Part model, mm, in its own coordinate system. Face numbers are marked on the shaded views. A direction names the side the tool comes from. Round coordinates to 2 decimals unless told otherwise and drop trailing zeros. Write each loop counter-clockwise with the first axis right and the second up, starting at its lowest first coordinate (ties: lowest second). Pieces come first, ordered by that corner, then holes. Notation, with made-up numbers: (35.25, 4.25) -> (80.25, 4.25) arc R17 cw to (80.25, 24.25) -> close; hole circle Ø6 at (87.5, 1.25). An arc over 180 degrees is marked (long way). Return JSON: item names as keys, results as strings. Group by question number.
```python
from build123d import *

# Parameters (mm, degrees)
SKETCH1_R                    = 4.572
SKETCH1_R_2                  = 1.397
SKETCH1_R_3                  = 3.175
BOSS_EXTRUDE1_DEPTH          = 6.35
F_3_8_0_375_DIAMETER_SLOT1_D = 9.525
SKETCH6_W                    = 9.906
SKETCH6_H                    = 38.1
BOSS_EXTRUDE2_DEPTH          = 76.2
SKETCH7_R                    = 1.397
SKETCH7_R_2                  = 1.7859375
CUT_EXTRUDE1_DEPTH           = 107.68
CUT_EXTRUDE2_DEPTH           = 10.16


with BuildPart() as part:
    # Sketch1 → Boss-Extrude1 (new body)
    with BuildSketch(Plane(origin=(0, 0, 0), x_dir=(1, 0, 0), z_dir=(0, 1, 0))):
        with BuildLine():
            Line((-53.34, 57.15), (53.34, 57.15))
            Line((53.34, 57.15), (53.34, -57.15))
            ThreePointArc((53.34, -57.15), (0, -110.49), (-53.34, -57.15))
            Line((-53.34, -57.15), (-53.34, 57.15))
        make_face()
        Circle(SKETCH1_R, mode=Mode.SUBTRACT)
        with Locations((-12.7, -12.7)):
            Circle(SKETCH1_R_2, mode=Mode.SUBTRACT)
        with Locations((-12.7, 12.7)):
            Circle(SKETCH1_R_2, mode=Mode.SUBTRACT)
        with Locations((12.7, 12.7)):
            Circle(SKETCH1_R_2, mode=Mode.SUBTRACT)
        with Locations((12.7, -12.7)):
            Circle(SKETCH1_R_2, mode=Mode.SUBTRACT)
        with Locations((0, -93.791156658)):
            Circle(SKETCH1_R_3, mode=Mode.SUBTRACT)
    extrude(amount=BOSS_EXTRUDE1_DEPTH)

    # 3/8 (0.375) Diameter Slot1 (through all)
    with Locations(Plane(origin=(0, 6.35, 0), x_dir=(1, 0, 0), z_dir=(0, 1, 0))):
        with Locations((0, 0)):
            Hole(F_3_8_0_375_DIAMETER_SLOT1_D / 2)

    # Sketch6 → Boss-Extrude2 (add)
    with BuildSketch(Plane(origin=(0, 6.35, 0), x_dir=(1, 0, 0), z_dir=(0, 1, 0))):
        with Locations((-48.387, 0)):
            Rectangle(SKETCH6_W, SKETCH6_H)
        with Locations((48.387, 0)):
            Rectangle(SKETCH6_W, SKETCH6_H)
    extrude(amount=BOSS_EXTRUDE2_DEPTH)

    # Sketch7 → Cut-Extrude1 (cut, through all)
    with BuildSketch(Plane.ZY.offset(53.34)):
        with Locations((-9.906, 63.455207007)):
            Circle(SKETCH7_R)
        with Locations((0, 63.5)):
            Circle(SKETCH7_R_2)
        with Locations((-7.036273203, 70.472926346)):
            Circle(SKETCH7_R)
        with Locations((-0.044792993, 73.406)):
            Circle(SKETCH7_R)
        with Locations((6.972926346, 70.536273203)):
            Circle(SKETCH7_R)
        with Locations((9.906, 63.544792993)):
            Circle(SKETCH7_R)
        with Locations((7.036273203, 56.527073654)):
            Circle(SKETCH7_R)
        with Locations((0.044792993, 53.594)):
            Circle(SKETCH7_R)
        with Locations((-6.972926346, 56.463726797)):
            Circle(SKETCH7_R)
    extrude(amount=-CUT_EXTRUDE1_DEPTH, mode=Mode.SUBTRACT)

    # Sketch8 → Cut-Extrude2 (cut)
    with BuildSketch(Plane(origin=(0, 6.35, 0), x_dir=(1, 0, 0), z_dir=(0, 1, 0))):
        Polygon((29.925449695, 49.207255953), (20.005730679, 57.103391791), (20.005730679, 41.311120115), align=None)
        Polygon((29.925449695, 49.207255953), (20.005730679, 41.311120115), (39.84516871, 41.311120115), align=None)
        Polygon((39.84516871, 41.311120115), (39.84516871, 57.103391791), (29.925449695, 49.207255953), align=None)
        Polygon((39.84516871, 57.103391791), (20.005730679, 57.103391791), (29.925449695, 49.207255953), align=None)
    extrude(amount=-CUT_EXTRUDE2_DEPTH, mode=Mode.SUBTRACT)


solid = part.part
```
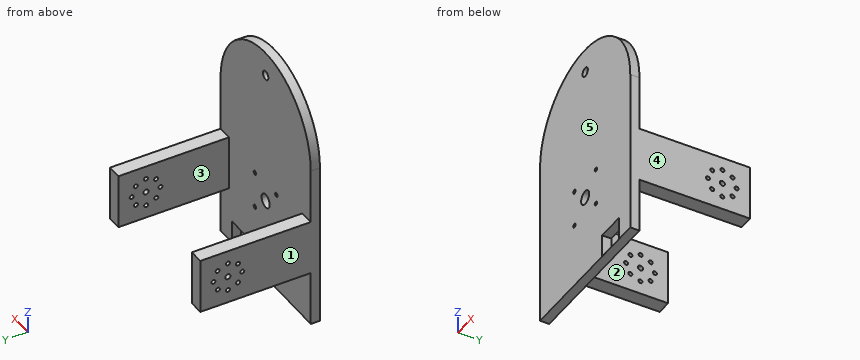
Item 1: Cut at B-B (y = 39.5). Write the cut outline in (x, z), then the cut area to 3 significant figures.
Item 2: Cut at D-D (x = -40). Write the cut outline in (y, z), then the cut area to 3 significant figures.
Item 3: Wall check: L1, parallel to Y at x = -46, z = 0; L2, parallel to X at y = 31, z = 3; L3, parallel to X at y = 4, z = 12. Give the ranges that are in metal, low to high.
Item 4: Two-plate mould, pull along X, no slides. Class the marked faces 3, 4 and 5: released by +X, released by -X, zero draft, split by the parting line, or undercut.
Item 5: Cut at C-C (z = -39). Write the cut outline in (x, y), then the cut area to 3 significant figures.
Item 6: Which spindle directions (+Z, -Z, +X, -X, +Y, -Y) get a long thin tool onto all of the face, cutting with end or side? Do the marked faces 1 and 2. Say none if no direction does.
Item 7: Cut at A-A (x = 0). Write the cut outline in (y, z), then the cut area to 3 significant figures.
Item 8: Flat gauge pins, fed straight in: P1, Ø8, axis at x = 46.5, y = 50.5, coming from the +Z side; P2, Ø12, axis at x = -4, y = 9, coming from the +Z side; P3, Ø1, axis at x = -27.5, z = 32.5, coming from the +Y side. Where does each tip first touch, or does it go through?
Checks:
{
 "1": {"outline": "(-53.34, -19.05) -> (-43.43, -19.05) -> (-43.43, 19.05) -> (-53.34, 19.05) -> close; (43.43, -19.05) -> (53.34, -19.05) -> (53.34, 19.05) -> (43.43, 19.05) -> close", "area": "755 mm2"},
 "2": {"outline": "(0, -57.15) -> (6.35, -57.15) -> (6.35, 92.44) -> (0, 92.44) -> close", "area": "950 mm2"},
 "3": {"L1": "y = 0 to 52.2, 54.99 to 61.71, 65.29 to 72.01, 74.8 to 82.55", "L2": "x = -53.34 to -43.43, 43.43 to 53.34", "L3": "x = -53.34 to -13.91, -11.49 to 11.49, 13.91 to 53.34"},
 "4": {"face 3": "undercut", "face 4": "released by +X", "face 5": "zero draft"},
 "5": {"outline": "(-53.34, 0) -> (53.34, 0) -> (53.34, 6.35) -> (-53.34, 6.35) -> close", "area": "677 mm2"},
 "6": {"face 1": "+Z, -Z, -X, +Y, -Y", "face 2": "+Z, -Z, +Y"},
 "7": {"outline": "(0, -57.15) -> (6.35, -57.15) -> (6.35, -4.76) -> (0, -4.76) -> close; (0, 4.76) -> (6.35, 4.76) -> (6.35, 90.62) -> (0, 90.62) -> close; (0, 96.97) -> (6.35, 96.97) -> (6.35, 110.49) -> (0, 110.49) -> close", "area": "964 mm2"},
 "8": {"P1": "stops at z = 19.05", "P2": "stops at z = 110.49", "P3": "stops at y = 6.35"}
}
